Source: CAD feature listing. Evaluate the final solid. Frame: model axes, mm. Face numbers are marked on the shaded views. Give positions to 0.01 mm unless a question says otherwise; leave off trailing zeros. Loops run counter-clockwise (first coordinate to the right, second up) from the corner with the lowest first, then second, coordinate; pieces in that order, holes last. Notation, with made-up numbers: (17.25, 72.25) -> (72.25, 72.25) arc R4 cw to (72.25, 79.25) -> close; hole circle Ø6 at (8, 44). An arc over 180 degrees is marked (long way). Return JSON: item names as keys, results as strings. Group by question number.
(1) Draft query along Z for the marked faces 1 and 2. Return one class per face: released by +Z, released by -Z, zero draft, split by the parting line, or undercut.
(2) Cut plane C-C on z = 1.8. Return loops of the section in (x, y) (3 decimals), then the cut area to 3 significant figures.
(3) Cut plane B-B on x = 0. Return loops of the section in (y, z) (3 decimals).
(4) Cut plane A-A on y = 0. Return loops of the section in (x, z) (3 decimals).
(5) Ray query, line 1 (X direction, y = -28.5, z = 1.65); line 2 (X direction, y = 30, z = 2.4); line 3 (Y direction, x = -12.7, z = 0.45). Return the intervals inside material, ascending. Write a range as from..to.
(6) Pin query (flat end, axial travel): pin 1 (1.5 mm diameter, centred on x = -28, z = 2, fed in from -Y); pin 2 (5 mm diameter, centred on x = -12.7, y = 27.98, fed in from +Z); pin 3 (1 mm diameter, centred on x = -12.5, z = 2.5, fed in from +Y). Return the tip coordinate at first contact, or that it passes through.
(7) Cut plane D-D on x = 28. Return loops of the section in (y, z) (3 decimals).
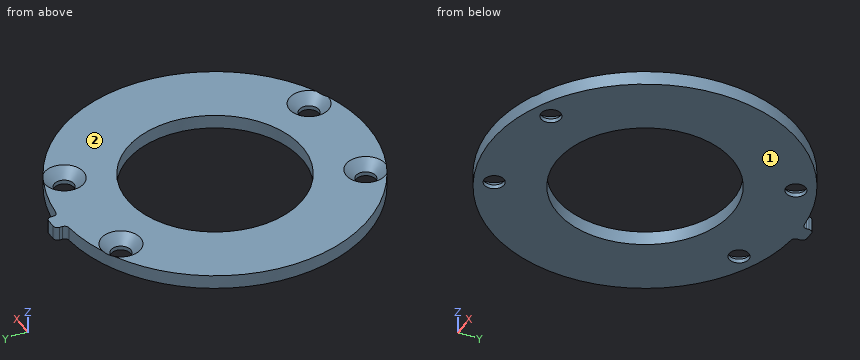
```python
from build123d import *

# Parameters (mm, degrees)
SKETCH2_R                    = 35
SKETCH2_R_2                  = 20
BOSS_EXTRUDE1_DEPTH          = 3.175
CSK_FOR_M4_SFHCS1_AT_2_COUNT = 2
CSK_FOR_M4_SFHCS1_AT_2_PITCH = 25.4
CSK_FOR_M4_SFHCS1_AT_3_COUNT = 2
CSK_FOR_M4_SFHCS1_AT_3_PITCH = 61.454142663
CSK_FOR_M4_SFHCS1_AT_4_COUNT = 2
CSK_FOR_M4_SFHCS1_AT_4_PITCH = 55.959375
SKETCH5_W                    = 4
SKETCH5_H                    = 5
BOSS_EXTRUDE2_DEPTH          = 3.175
FILLET1_R                    = 1


with BuildPart() as part:
    # Sketch2 → Boss-Extrude1 (new body)
    with BuildSketch(Plane.XY):
        Circle(SKETCH2_R)
        Circle(SKETCH2_R_2, mode=Mode.SUBTRACT)
    extrude(amount=BOSS_EXTRUDE1_DEPTH)

    # Sketch4 → CSK for M4 SFHCS1 (revolve, cut)
    with BuildSketch(Plane(origin=(-12.7, 27.9796875, 3.175), x_dir=(0, -1, 0), z_dir=(1, 0, 0))):
        Polygon((0, 0), (0, 3.175), (2.25, 3.175), (2.25, 2.23), (4.48, 0), align=None)
    csk_for_m4_sfhcs1 = revolve(axis=Axis((-12.7, 27.9796875, 9.525), (0, 0, -1)), mode=Mode.SUBTRACT)

    # CSK for M4 SFHCS1 at 2: CSK for M4 SFHCS1 ×2
    with Locations(*[(i * CSK_FOR_M4_SFHCS1_AT_2_PITCH, 0, 0) for i in range(1, CSK_FOR_M4_SFHCS1_AT_2_COUNT)]):
        add(csk_for_m4_sfhcs1, mode=Mode.SUBTRACT)

    # CSK for M4 SFHCS1 at 3: CSK for M4 SFHCS1 ×2
    with Locations(*[Vector(0.413316318, -0.910587514, 0) * (i * CSK_FOR_M4_SFHCS1_AT_3_PITCH) for i in range(1, CSK_FOR_M4_SFHCS1_AT_3_COUNT)]):
        add(csk_for_m4_sfhcs1, mode=Mode.SUBTRACT)

    # CSK for M4 SFHCS1 at 4: CSK for M4 SFHCS1 ×2
    with Locations(*[(0, -i * CSK_FOR_M4_SFHCS1_AT_4_PITCH, 0) for i in range(1, CSK_FOR_M4_SFHCS1_AT_4_COUNT)]):
        add(csk_for_m4_sfhcs1, mode=Mode.SUBTRACT)

    # Sketch5 → Boss-Extrude2 (add)
    with BuildSketch(Plane(origin=(0, 0, 0), x_dir=(-1, 0, 0), z_dir=(0, 0, -1))):
        with Locations((0, 35)):
            Rectangle(SKETCH5_W, SKETCH5_H)
    extrude(amount=-BOSS_EXTRUDE2_DEPTH)

    # Fillet1
    fillet1_edges = [part.edges().sort_by_distance(p)[0] for p in [
        (-2, 37.5, 1.5875),
        (-2, 34.942810419, 1.5875),
        (2, 37.5, 1.5875),
        (2, 34.942810419, 1.5875),
    ]]
    fillet(fillet1_edges, radius=FILLET1_R)


solid = part.part
```
Answers:
{
 "1": {"face 1": "released by -Z", "face 2": "released by +Z"},
 "2": {"outline": "(-2.917, 34.878) arc R35 ccw (long way) to (2.917, 34.878) arc R1 cw to (2, 35.875) -> (2, 36.5) arc R1 ccw to (1, 37.5) -> (-1, 37.5) arc R1 ccw to (-2, 36.5) -> (-2, 35.875) arc R1 cw to start; hole circle Ø40 at (0, 0); hole circle Ø6.21 at (-12.7, -27.98); hole circle Ø6.21 at (-12.7, 27.98); hole circle Ø6.21 at (12.7, -27.98); hole circle Ø6.21 at (12.7, 27.98)", "area": "2,480 mm²"},
 "3": {"outline": "(-35, 0) -> (-20, 0) -> (-20, 3.175) -> (-35, 3.175) -> close; (20, 0) -> (37.5, 0) -> (37.5, 3.175) -> (20, 3.175) -> close"},
 "4": {"outline": "(-35, 0) -> (-20, 0) -> (-20, 3.175) -> (-35, 3.175) -> close; (20, 0) -> (35, 0) -> (35, 3.175) -> (20, 3.175) -> close"},
 "5": {"line 1": "-20.32..-15.61, -9.79..9.79, 15.61..20.32", "line 2": "-18.03..-15.81, -9.59..9.59, 15.81..18.03", "line 3": "-32.61..-30.23, -25.73..-15.45, 15.45..25.73, 30.23..32.61"},
 "6": {"pin 1": "y = -21.96", "pin 2": "z = 1.2", "pin 3": "y = 32.88"},
 "7": {"outline": "(-21, 0) -> (21, 0) -> (21, 3.175) -> (-21, 3.175) -> close"}
}
